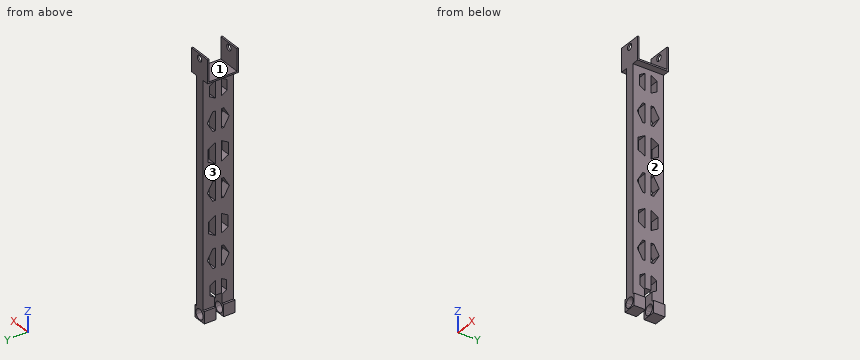
from build123d import *

# Parameters (mm, degrees)
SKETCH_1_W                      = 6
SKETCH_1_H                      = 20
EXTRUDE_1_DEPTH                 = 165
HOLE_WIZARD_G1_16_1_D           = 6.6
HOLE_WIZARD_G1_16_1_DEPTH       = 50
HOLE_WIZARD_G1_16_1_CSINK_D     = 7.773
HOLE_WIZARD_G1_16_1_CSINK_ANGLE = 90
HOLE_WIZARD_G1_16_1_TIP         = 1.982840043
SKETCH_5_W                      = 15
SKETCH_5_H                      = 20
EXTRUDE_2_DEPTH                 = 10
EXTRUDE_2_DEPTH_BACK            = 15
SKETCH_6_W                      = 5.5
SKETCH_6_H                      = 15
SKETCH_6_W_2                    = 4.5
CUT_EXTRUDE_1_DEPTH             = 32
SKETCH_7_W                      = 15
SKETCH_7_H                      = 18
CUT_EXTRUDE_2_DEPTH             = 14
SKETCH_8_R                      = 2
CUT_EXTRUDE_3_DEPTH             = 39
CUT_EXTRUDE_4_DEPTH             = 70
EXTRUDE_3_DEPTH                 = 20
SKETCH_11_5_W                   = 6
SKETCH_11_5_H                   = 1.141567996
CUT_EXTRUDE_5_DEPTH             = 20
CUT_EXTRUDE_6_DEPTH             = 20


with BuildPart() as part:
    # Sketch 1 → Extrude 1 (new body)
    with BuildSketch(Plane.XY):
        Rectangle(SKETCH_1_W, SKETCH_1_H)
    extrude(amount=EXTRUDE_1_DEPTH)

    # Hole Wizard G1_16 _1
    with Locations(Plane(origin=(3, 0, 0), x_dir=(0, 0, -1), z_dir=(1, 0, 0))):
        with Locations((-5, 0)):
            CounterSinkHole(HOLE_WIZARD_G1_16_1_D / 2, HOLE_WIZARD_G1_16_1_CSINK_D / 2, depth=HOLE_WIZARD_G1_16_1_DEPTH, counter_sink_angle=HOLE_WIZARD_G1_16_1_CSINK_ANGLE)
            with Locations((0, 0, -(HOLE_WIZARD_G1_16_1_DEPTH + HOLE_WIZARD_G1_16_1_TIP / 2))):  # 118° drill point
                Cone(0, HOLE_WIZARD_G1_16_1_D / 2, HOLE_WIZARD_G1_16_1_TIP, mode=Mode.SUBTRACT)

    # Sketch 5 → Extrude 2 (add, two sides)
    with BuildSketch(Plane(origin=(3, 0, 0), x_dir=(0, 0, -1), z_dir=(1, 0, 0))) as extrude_2_sk:
        with Locations((-160.5, 0)):
            Rectangle(SKETCH_5_W, SKETCH_5_H)
    extrude(amount=EXTRUDE_2_DEPTH)
    extrude(extrude_2_sk.sketch, amount=-EXTRUDE_2_DEPTH_BACK)

    # Sketch 6 → Cut-Extrude 1 (cut)
    with BuildSketch(Plane.XZ.offset(10)):
        with Locations((10.25, 160.5)):
            Rectangle(SKETCH_6_W, SKETCH_6_H)
        with Locations((-9.75, 160.5)):
            Rectangle(SKETCH_6_W_2, SKETCH_6_H)
    extrude(amount=-CUT_EXTRUDE_1_DEPTH, mode=Mode.SUBTRACT)

    # Sketch 7 → Cut-Extrude 2 (cut)
    with BuildSketch(Plane.XY.offset(168)):
        Rectangle(SKETCH_7_W, SKETCH_7_H)
    extrude(amount=-CUT_EXTRUDE_2_DEPTH, mode=Mode.SUBTRACT)

    # Sketch 8 → Cut-Extrude 3 (cut)
    with BuildSketch(Plane(origin=(0, 10, 0), x_dir=(1, 0, 0), z_dir=(0, 1, 0))):
        with Locations((0, -165)):
            Circle(SKETCH_8_R)
    extrude(amount=-CUT_EXTRUDE_3_DEPTH, mode=Mode.SUBTRACT)

    # Sketch 9 → Cut-Extrude 4 (cut)
    with BuildSketch(Plane.ZY.offset(3)):
        Polygon((14.328441006, 1.918732887), (24.619003084, 1.918732887), (22.600253038, 5.415310533), (16.347191051, 5.415310533), align=None)
        Polygon((22.600253038, -5.415310533), (24.57465807, -1.995540703), (14.372786019, -1.995540703), (16.347191051, -5.415310533), align=None)
        Polygon((32.73389091, 1.918732887), (45.062363825, 1.918732887), (45.062363825, 3.558923578), (38.898127367, 7.117847156), (32.73389091, 3.558923578), align=None)
        Polygon((45.062363825, -3.558923578), (45.062363825, -1.995540703), (32.73389091, -1.995540703), (32.73389091, -3.558923578), (38.898127367, -7.117847156), align=None)
        Polygon((52.911163907, 1.918732887), (65.330427938, 1.918732887), (62.779502404, 6.337065517), (55.46208944, 6.337065517), align=None)
        Polygon((62.779502404, -6.337065517), (65.286082924, -1.995540703), (52.95550892, -1.995540703), (55.46208944, -6.337065517), align=None)
        Polygon((87.237271272, -3.558923578), (87.237271272, -1.995540703), (74.908798357, -1.995540703), (74.908798357, -3.558923578), (81.073034814, -7.117847156), align=None)
        Polygon((74.908798357, 1.918732887), (87.237271272, 1.918732887), (87.237271272, 3.558923578), (81.073034814, 7.117847156), (74.908798357, 3.558923578), align=None)
        Polygon((97.746948796, 1.918732887), (110.964476059, 1.918732887), (108.213984717, 6.682723636), (100.497440137, 6.682723636), align=None)
        Polygon((108.213984717, -6.682723636), (110.920131045, -1.995540703), (97.791293809, -1.995540703), (100.497440137, -6.682723636), align=None)
        Polygon((118.547188397, 1.918732887), (130.875661312, 1.918732887), (130.875661312, 3.558923578), (124.711424854, 7.117847156), (118.547188397, 3.558923578), align=None)
        Polygon((130.875661312, -3.558923578), (130.875661312, -1.995540703), (118.547188397, -1.995540703), (118.547188397, -3.558923578), (124.711424854, -7.117847156), align=None)
        Polygon((138.857505266, 1.918732887), (149.946330576, 1.918732887), (147.728014723, 5.760968652), (141.075821119, 5.760968652), align=None)
        Polygon((147.728014723, -5.760968652), (149.901985563, -1.995540703), (138.901850279, -1.995540703), (141.075821119, -5.760968652), align=None)
    extrude(amount=-CUT_EXTRUDE_4_DEPTH, mode=Mode.SUBTRACT)

    # Sketch 11 → Extrude 3 (add)
    with BuildSketch(Plane(origin=(0, -10, 0), x_dir=(-1, 0, 0), z_dir=(0, -1, 0))):
        with BuildLine():
            Line((-3, -3.625227292), (-3, -1.141567996))
            Line((-3, -1.141567996), (-4.178650157, -1.141567996))
            Line((-4.178650157, -1.141567996), (-4.178650157, -8.860192338))
            Line((-4.178650157, -8.860192338), (-3, -8.860192338))
            Line((-3, -8.860192338), (-3, -6.374772708))
            ThreePointArc((-3, -6.374772708), (-3.3, -5), (-3, -3.625227292))
        make_face()
        with BuildLine():
            Line((4.356093251, -8.860192338), (4.356093251, -1.141567996))
            Line((4.356093251, -1.141567996), (3, -1.141567996))
            Line((3, -1.141567996), (3, -3.625227292))
            ThreePointArc((3, -3.625227292), (3.224127789, -4.296437636), (3.3, -5))
            ThreePointArc((3.3, -5), (3.224127789, -5.703562364), (3, -6.374772708))
            Line((3, -6.374772708), (3, -8.860192338))
            Line((3, -8.860192338), (4.356093251, -8.860192338))
        make_face()
        with BuildLine():
            Line((3, -3.625227292), (3, -1.141567996))
            Line((3, -1.141567996), (-3, -1.141567996))
            Line((-3, -1.141567996), (-3, -3.625227292))
            ThreePointArc((-3, -3.625227292), (0, -1.7), (3, -3.625227292))
        make_face()
        with BuildLine():
            Line((-3, -8.860192338), (3, -8.860192338))
            Line((3, -8.860192338), (3, -6.374772708))
            ThreePointArc((3, -6.374772708), (0, -8.3), (-3, -6.374772708))
            Line((-3, -6.374772708), (-3, -8.860192338))
        make_face()
    extrude(amount=-EXTRUDE_3_DEPTH)

    # Sketch 11_5 → Cut-Extrude 5 (cut)
    with BuildSketch(Plane(origin=(0, -10, 0), x_dir=(-1, 0, 0), z_dir=(0, -1, 0))):
        with Locations((0, -0.570783998)):
            Rectangle(SKETCH_11_5_W, SKETCH_11_5_H)
        with BuildLine():
            Line((3, -6.374772708), (3, -3.625227292))
            ThreePointArc((3, -3.625227292), (0, -1.7), (-3, -3.625227292))
            Line((-3, -3.625227292), (-3, -6.374772708))
            ThreePointArc((-3, -6.374772708), (0, -8.3), (3, -6.374772708))
        make_face()
    extrude(amount=-CUT_EXTRUDE_5_DEPTH, mode=Mode.SUBTRACT)

    # Sketch 13 → Cut-Extrude 6 (cut)
    with BuildSketch(Plane(origin=(4.178650157, 0, 0), x_dir=(0, 0, -1), z_dir=(1, 0, 0))):
        Polygon((-8.858432004, -2.55), (-1.141567996, -2.55), (-1.141567996, 2.55), (-8.858432004, 2.55), (-15.473063701, 2.55), (-15.473063701, -2.55), align=None)
    extrude(amount=-CUT_EXTRUDE_6_DEPTH, mode=Mode.SUBTRACT)


solid = part.part
Work out the finished part from the listing and answer in its coordinate system (mm). Face numbers are marked on the shaded views. Round coordinates to 2 decimals unless told otherwise and drop trailing zeros. Order: outer loops, then holes, each group sorted by start corner. A loop starts at its lowest first (then second) coordinate and runs counter-clockwise, first axis right, second up. Notation, with made-up numbers: M -35,7 L -23,7 A21 cw -23,40 Z; hole C -20.75,1 d3. An arc over 180 degrees is marked long. Put each result on its own line as item: value. Start each with the question number.
Q1. Section B-B, the plane x = 0 is taken. Give the number of separate pieces and of enclosed holes in the cut face, and give its area (3 significant figures).
Q2. Section C-C, the plane z = 135.5 is taken. Write down the section's boundary in (x, y), and give its area (3 significant figures).
Q3. Straight lines are drawn through the part: L1, parallel to Z at x = 0, y = 9.4; L2, parallel to Y at x = -1.25, z = 106.5; L3, parallel to Y at x = -0.5, z = 123. For each, find the intervals that lie inside material, in ascending order. Write a range as [from, to].
Q4. Flat-ended cylindrical pins translate along their axes: pin 1 (2 mm diameter, centred on y = 6, z = 3, fed in from +X); pin 2 (3 mm diameter, centred on x = 5.5, z = 151, fed in from +Y); pin 3 (4 mm diameter, centred on y = -6, z = 143, fed in from -X); pin 4 (2 mm diameter, centred on y = 7, z = 101, fed in from +X). Find the tip coordinate at first contact, or state that the pin passes through.
Q5. For a pull along Z with two mould halves and no side action, classify the marked faces 1, 2 and 3 as pulls with the +Z half, pulls with the -Z half, needs draft (parallel to the pull), parting line crosses it, or undercut.
Q6. Section A-A, the plane z = 165 is taken. Write down the section's boundary in (x, y).
Findings below:
1. separate pieces: 5
1. enclosed holes: 12
1. area: 2,350 mm^2
2. outline: M -3,-10 L 3,-10 L 3,10 L -3,10 Z
2. area: 120 mm^2
3. L1: z = [1.14, 1.7], [8.3, 163], [167, 168]
3. L2: y = [-10, -6.68], [-2, 1.92], [6.68, 10]
3. L3: y = [-10, -6.13], [-2, 1.92], [6.13, 10]
4. pin 1: stops at x = 4.18
4. pin 2: passes through
4. pin 3: stops at x = -3
4. pin 4: stops at x = 3
5. face 1: pulls with the +Z half
5. face 2: undercut
5. face 3: undercut
6. outline: M -7.5,-10 L -2,-10 L -2,-9 L -7.5,-9 Z; M -7.5,9 L -2,9 L -2,10 L -7.5,10 Z; M 2,-10 L 7.5,-10 L 7.5,-9 L 2,-9 Z; M 2,9 L 7.5,9 L 7.5,10 L 2,10 Z
